```python
from build123d import *

# Parameters (mm, degrees)
DODANIE_WYCI_GNI_CIE1_DEPTH                       = 8
WYTNIJ_WYCI_GNI_CIE1_DEPTH                        = 8
WYTNIJ_WYCI_GNI_CIE2_DEPTH                        = 39.404607438
WYTNIJ_WYCI_GNI_CIE2_DEPTH_BACK                   = 39.404607438
POG_BIENIE_WALCOWE_POD_M5_RUB_Z_BEM_W_D           = 5.3
POG_BIENIE_WALCOWE_POD_M5_RUB_Z_BEM_W_CBORE_D     = 10
POG_BIENIE_WALCOWE_POD_M5_RUB_Z_BEM_W_CBORE_DEPTH = 5
ZAOKR_GLENIE1_R                                   = 3
ZAOKR_GLENIE2_R                                   = 1


with BuildPart() as part:
    # Szkic1 → Dodanie-wyciągnięcie1 (new, symmetric)
    with BuildSketch(Plane.XY):
        Polygon((0, 0), (28.58974359, 0), (31.794871795, 20), (0, 20), align=None)
    dodanie_wyci_gni_cie1 = extrude(amount=DODANIE_WYCI_GNI_CIE1_DEPTH, both=True)

    # Lustro1: Dodanie-wyciągnięcie1 across plane
    add(dodanie_wyci_gni_cie1.mirror(Plane(origin=(0, 20, 8), x_dir=(0, 0, 1), z_dir=(1, 0, 0))))

    # Szkic2 → Wytnij-wyciągnięcie1 (cut)
    with BuildSketch(Plane.XY.offset(8)):
        with BuildLine():
            Line((-13, 20), (13, 20))
            ThreePointArc((13, 20), (0, 7), (-13, 20))
        make_face()
    extrude(amount=-WYTNIJ_WYCI_GNI_CIE1_DEPTH, mode=Mode.SUBTRACT)

    # Szkic3 → Wytnij-wyciągnięcie2 (cut, two sides: drawn at the far end of the back side and taken through both)
    with BuildSketch(Plane.XY.offset(-WYTNIJ_WYCI_GNI_CIE2_DEPTH_BACK)):
        with BuildLine():
            ThreePointArc((-9, 20), (0, 11), (9, 20))
            Line((9, 20), (-9, 20))
        make_face()
    extrude(amount=WYTNIJ_WYCI_GNI_CIE2_DEPTH + WYTNIJ_WYCI_GNI_CIE2_DEPTH_BACK, mode=Mode.SUBTRACT)

    # Pogłębienie walcowe pod M5 Śrubę z łbem walcowym z gniazdem1 (through all)
    with Locations(Plane(origin=(0, 0, 0), x_dir=(-1, 0, 0), z_dir=(0, -1, 0))):
        with Locations((-17.5, 0), (17.5, 0)):
            CounterBoreHole(POG_BIENIE_WALCOWE_POD_M5_RUB_Z_BEM_W_D / 2, POG_BIENIE_WALCOWE_POD_M5_RUB_Z_BEM_W_CBORE_D / 2, POG_BIENIE_WALCOWE_POD_M5_RUB_Z_BEM_W_CBORE_DEPTH)

    # Zaokrąglenie1
    zaokr_glenie1_edges = [part.edges().sort_by_distance(p)[0] for p in [
        (-28.58974359, 0, 0),
        (28.58974359, 0, 0),
    ]]
    fillet(zaokr_glenie1_edges, radius=ZAOKR_GLENIE1_R)

    # Zaokrąglenie2
    zaokr_glenie2_edges = [part.edges().sort_by_distance(p)[0] for p in [
        (0, 11, 0),
        (0, 11, -8),
        (0, 0, -8),
        (0, 0, 8),
        (30.394654482, 11.262643966, -8),
        (-30.394654482, 11.262643966, -8),
        (27.978494862, 0.717004577, -8),
        (-27.978494862, 0.717004577, -8),
        (-30.394654482, 11.262643966, 8),
        (30.394654482, 11.262643966, 8),
        (27.978494862, 0.717004577, 8),
        (-27.978494862, 0.717004577, 8),
    ]]
    fillet(zaokr_glenie2_edges, radius=ZAOKR_GLENIE2_R)


solid = part.part
```
The model under review builds one solid part; all positions refer to its coordinate system, in mm. A direction names the side the tool comes from. Give positions to 0.01 mm unless a question says otherwise; leave off trailing zeros. Write each loop counter-clockwise with the first axis right and the second up, starting at its lowest first coordinate (ties: lowest second). Pieces come first, ordered by that corner, then holes. Notation, with made-up numbers: (-19, 29.25) - (19, 29.25) arc R17 cw to (19, 40.25) - close; hole circle Ø3 at (-33, 69). An arc over 180 degrees is marked (long way). Answer in a Markdown table with one row per item. Add a question column.
1. Insertion check: P1, Ø8.5, axis at x = -17.5, z = 0, coming from the +Y side; P2, Ø5, axis at x = 6.5, y = 14.5, coming from the +Z side; P3, Ø3, axis at x = -17, z = -1, coming from the -Y side; P4, Ø1, axis at y = 11.5, z = 0.5, coming from the -X side. Each pin has a flat end and moves straight along its axis. Give the tip position at first contact, or say it passes through.
2. We need section B-B on z = 6.25. Write out the cut boundary in (x, y).
3. We need section C-C on y = 11.75. State how many separate pieces and enclosed holes the cut face has, then the cut area to 3 significant figures.
4. We need section A-A on x = 17.5. Write out the cut boundary in (y, z), then the cut area to 3 significant figures.
5. Tool access review of faces 1 (the cylindrical face through (-30.13, 11.43, 7.7)), 2 (the flat face through (-20, 5, 2)), 3 (the flat face through (0.1, 9.7, 0)): name each direction out of +Z, -Z, +X, -X, +Y, -Y from which nothing blocks a thin tool from reaching the whole face with its end or side.
6. Draft analysis for pull direction Z (two halves, no side actions). For faces 4 (the flat face through (0, 6, 8)), 5 (the cylindrical face through (-12.505, 2.465, -0.22)), 6 (the cylindrical face through (-30.093, 11.185, -7.699)), state which applies: +Z half, -Z half, draft (parallel to the pull), parting line (faces both ways), or undercut.
7. Wall thickness on line 1 along X through (y, z) = (1.25, -2.75); line 2 along Z through (x, y) = (-17.5, 1.35); line 3 along Y through (x, z) = (-17, 4.25): over which ranges is each line inside the solid? List them lowest first. Write a range as [from, to].
8. We need section D-D on x = 0. Write out the cut boundary in (y, z).
Ans:
| question | item | result |
|---|---|---|
| 1 | P1 | stops at y = 20 |
| 1 | P2 | stops at z = 0 |
| 1 | P3 | passes through |
| 1 | P4 | stops at x = -30.51 |
| 2 | outline | (-31.79, 20) - (-28.99, 2.53) arc R3 ccw to (-26.03, 0) - (26.03, 0) arc R3 ccw to (28.99, 2.53) - (31.79, 20) - (13, 20) arc R13 cw to (-13, 20) - close |
| 3 | separate pieces | 2 |
| 3 | enclosed holes | 2 |
| 3 | area | 710 mm^2 |
| 4 | outline | (0, -7) arc R1 ccw to (1, -8) - (20, -8) - (20, -2.65) - (5, -2.65) - (5, -5) - (0, -5) - close; (0, 5) - (5, 5) - (5, 2.65) - (20, 2.65) - (20, 8) - (1, 8) arc R1 ccw to (0, 7) - close |
| 4 | area | 190 mm^2 |
| 5 | face 1 | +Z, -X, -Y |
| 5 | face 2 | -Y |
| 5 | face 3 | +Z, +Y |
| 6 | face 4 | +Z half |
| 6 | face 5 | undercut |
| 6 | face 6 | -Z half |
| 7 | line 1 | x = [-28.47, -21.68], [-13.32, 13.32], [21.68, 28.47] |
| 7 | line 2 | z = [-8, -5], [5, 8] |
| 7 | line 3 | y = [5, 20] |
| 8 | outline | (0, -7) arc R1 ccw to (1, -8) - (10, -8) arc R1 ccw to (11, -7) - (11, -1) arc R1 ccw to (10, 0) - (7, 0) - (7, 8) - (1, 8) arc R1 ccw to (0, 7) - close |
